```python
from build123d import *

# Parameters (mm, degrees)
CYLINDER031_R     = 3
CYLINDER031_DEPTH = 21
BOX006_W          = 21
BOX006_H          = 25
BOX006_DEPTH      = 4
CYLINDER026_R     = 1.5
CYLINDER026_DEPTH = 52
CYLINDER021_R     = 3
CYLINDER021_DEPTH = 30
CYLINDER032_R     = 5
CYLINDER032_DEPTH = 6


with BuildPart() as cylindre027:
    # Cylinder031 → Cylinder031 (new body)
    with BuildSketch(Plane(origin=(3, 19, -161), x_dir=(1, 0, 0), z_dir=(0, 0, 1))):
        Circle(CYLINDER031_R)
    extrude(amount=CYLINDER031_DEPTH)


with BuildPart() as cube006:
    # Box006 → Box006 (new body)
    with BuildSketch(Plane(origin=(-9, 7, -140), x_dir=(1, 0, 0), z_dir=(0, 0, 1))):
        with Locations((10.5, 12.5)):
            Rectangle(BOX006_W, BOX006_H)
    extrude(amount=BOX006_DEPTH)


with BuildPart() as cylindre022:
    # Cylinder026 → Cylinder026 (new body)
    with BuildSketch(Plane(origin=(-26, 6, -138), x_dir=(0, 0, -1), z_dir=(1, 0, 0))):
        Circle(CYLINDER026_R)
    extrude(amount=CYLINDER026_DEPTH)


with BuildPart() as fusion006:
    # Cylinder021 → Cylinder021 (new body)
    with BuildSketch(Plane(origin=(-13, 6, -138), x_dir=(0, 0, -1), z_dir=(1, 0, 0))):
        Circle(CYLINDER021_R)
    extrude(amount=CYLINDER021_DEPTH)

    # Cut019: cut Cylindre022
    add(cylindre022.part, mode=Mode.SUBTRACT)


with BuildPart() as fusion006_1:
    # Cut019 placement: moved
    add(fusion006.part.moved(Location((0, -1, 0))))

    # Fusion005: union Cube006
    add(cube006.part)

    # Fusion006: union Cylindre027
    add(cylindre027.part)


with BuildPart() as obj1:
    # Cylinder032 → Cylinder032 (new body)
    with BuildSketch(Plane(origin=(3, 19, -165), x_dir=(1, 0, 0), z_dir=(0, 0, 1))):
        Circle(CYLINDER032_R)
    extrude(amount=CYLINDER032_DEPTH)

    # Fusion007: union Fusion006
    add(fusion006_1.part)


with BuildPart() as obj1_1:
    # Fusion007 placement: moved
    add(obj1.part.moved(Location((-2.5, 0, 0))))


solid = obj1_1.part
```
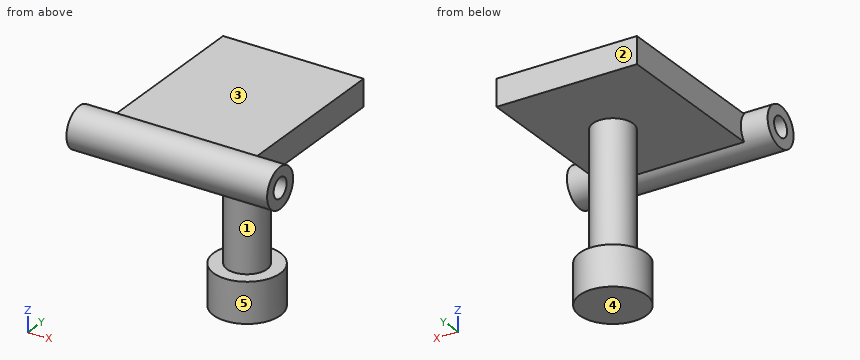
Can you work these out from the model? Positions are in its coordinate system, mm. Face numbers are marked on the shaded views. A direction names the side the tool comes from. Coordinates: 2 decimals unless noted, no trailing zeros. Loops run counter-clockwise (first coordinate to the right, second up) from the corner with the lowest first, then second, coordinate; pieces in that order, holes last.
1) I need wall thicknesses on probe 1 along Y at (x, z) = (8.75, -138); probe 2 along Z at (x, y) = (-5.5, 15.25); probe 3 along Z at (x, y) = (0.25, 15.25). Which ranges of each line are inside material? Lowest first, please.
2) Which directions (+Z, -Z, +X, -X, +Y, -Y) give clear straight access to the entire face, cutting with the end or side of a thin tool? Please do the marked faces 4 and 5.
3) Imagine slicing it at B-B on y = 5. List the corners of the cut face in (x, z) for me, plus the area to 3 significant figures.
4) Imagine slicing it at D-D on x = -4. List the corners of the cut face in (y, z) for me, plus the area to 3 significant figures.
5) Thinking about a two-plate mould opening in Z: for the marked faces 1, 2 and 3, which applies, pulls with the +Z half, pulls with the -Z half, needs draft (parallel to the pull), parting line crosses it, or undercut?
6) For pin 1 (3 mm diameter, centred on y = 21, z = -138.5, fed in from +X); pin 2 (8 mm diameter, centred on y = 21, z = -159, fed in from -X); pin 3 (10.5 mm diameter, centred on x = -4.5, y = 14.5, fed in from +Z), each with a flat end and sliding along its axis, tell me the tip position at first contact or that it passes through.
7) Imagine slicing it at C-C on x = 0.5. List the corners of the cut face in (y, z) for me.
8) Imagine slicing it at A-A on z = -138. List the corners of the cut face in (x, y) for me.
Completed:
1. probe 1: y = 2 to 3.5, 6.5 to 32
1. probe 2: z = -140 to -136
1. probe 3: z = -165 to -159, -140 to -136
2. face 4: -Z, +X, -X, +Y, -Y
2. face 5: -Z
3. outline: (-15.5, -141) - (14.5, -141) - (14.5, -139.5) - (-15.5, -139.5) - close; (-15.5, -136.5) - (14.5, -136.5) - (14.5, -135) - (-15.5, -135) - close
3. area: 90.0 mm2
4. outline: (7.24, -140) - (32, -140) - (32, -136) - (7.24, -136) arc R3 ccw (long way) to start; (16.82, -165) - (21.18, -165) - (21.18, -159) - (16.82, -159) - close; hole circle Ø3 at (5, -138)
4. area: 144 mm2
5. face 1: undercut
5. face 2: needs draft
5. face 3: pulls with the +Z half
6. pin 1: stops at x = 9.5
6. pin 2: stops at x = -4.5
6. pin 3: stops at z = -136
7. outline: (7.24, -140) - (16, -140) - (16, -159) - (14, -159) - (14, -165) - (24, -165) - (24, -159) - (22, -159) - (22, -140) - (32, -140) - (32, -136) - (7.24, -136) arc R3 ccw (long way) to start; hole circle Ø3 at (5, -138)
8. outline: (-15.5, 2) - (14.5, 2) - (14.5, 3.5) - (-15.5, 3.5) - close; (-15.5, 6.5) - (14.5, 6.5) - (14.5, 8) - (9.5, 8) - (9.5, 32) - (-11.5, 32) - (-11.5, 8) - (-15.5, 8) - close
